Verification items for the finished model (mm, model axes). Face numbers are marked on the shaded views. A direction names the side the tool comes from. Give positions to 0.01 mm unless a question says otherwise; leave off trailing zeros. Write each loop counter-clockwise with the first axis right and the second up, starting at its lowest first coordinate (ties: lowest second). Pieces come first, ordered by that corner, then holes. Notation, with made-up numbers: (40, -20.5) - (57, -20.5) arc R9 cw to (57, -15.5) - close; hole circle Ø6 at (69, 38). An arc over 180 degrees is marked (long way). Answer as a JSON object with one key per item and string values. Group by question number.
Item 1: Sectioned sample at C-C, the plane y = -4.75. Record the boundary of the cut face in (x, z).
Item 2: Draft check along Y on the marked faces 4, 5, 6 and 7. Enter one of: +Y half, -Y half, draft (parallel to the pull), parting line (faces both ways), or undercut.
Item 3: Sectioned sample at A-A, the plane x = -9. Record the boundary of the cut face in (y, z).
Item 4: Sectioned sample at B-B, the plane z = 33. Record the boundary of the cut face in (x, y), and give its area (3 significant figures).
Item 5: Tool access check on the marked faces 1, 2 and 3. Record the directions out of +Z, -Z, +X, -X, +Y, -Y that give a thin tool (end or side, any length) a straight path to the whole face; none if there is none.
Item 6: Scan lines: line 1 along X through (y, z) = (-1.25, 44.5); line 2 along Y through (x, z) = (-0.5, 53.5); line 3 along X through (y, z) = (-7.25, 35). Record each from-to range of solid material in increasing order. Write a range as [from, to].
Item 7: Go/stop test with flat-tipped pins: pin 1 (0.9 mm diameter, centred on y = 8, z = 33.5, fed in from -X); pin 2 (0.9 mm diameter, centred on y = 8.5, z = 37, fed in from +X). Record where each tip stops, or that it passes through.
Item 8: Sectioned sample at D-D, the plane z = 53. Record the boundary of the cut face in (x, y).
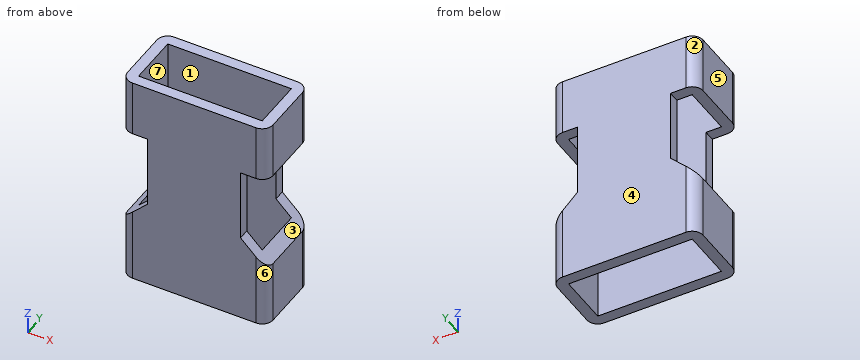
```python
from build123d import *

# Parameters (mm, degrees)
F0_W     = 34
F0_H     = 14
F1_DEPTH = 60
F3_DEPTH = 12.5


with BuildPart() as f1:
    # F0 (on Top) → F1 (new body)
    with BuildSketch(Plane.XY):
        with BuildLine():
            Line((-17, -10), (17, -10))
            ThreePointArc((17, -10), (19.12132, -9.12132), (20, -7))
            Line((20, -7), (20, 7))
            ThreePointArc((20, 7), (19.12132, 9.12132), (17, 10))
            Line((17, 10), (-17, 10))
            ThreePointArc((-17, 10), (-19.12132, 9.12132), (-20, 7))
            Line((-20, 7), (-20, -7))
            ThreePointArc((-20, -7), (-19.12132, -9.12132), (-17, -10))
        make_face()
        Rectangle(F0_W, F0_H, mode=Mode.SUBTRACT)
    extrude(amount=F1_DEPTH)

    # F2 (on Front) → F3 (cut, symmetric)
    with BuildSketch(Plane.XZ):
        Polygon((-25.043013, 44.406913), (-22.849802, 14.579257), (-12.761037, 24.448702), (-12.761037, 44.406913), align=None)
        Polygon((22.849802, 14.579257), (25.043013, 44.406913), (12.761037, 44.406913), (12.761037, 24.448702), align=None)
    extrude(amount=F3_DEPTH, both=True, mode=Mode.SUBTRACT)


solid = f1.part
```
Geometry check:
{
 "1": {"outline": "(-20, 0) - (-17, 0) - (-17, 20.3) - (-20, 17.37) - close; (-20, 44.41) - (-17, 44.41) - (-17, 60) - (-20, 60) - close; (17, 0) - (20, 0) - (20, 17.37) - (17, 20.3) - close; (17, 44.41) - (20, 44.41) - (20, 60) - (17, 60) - close"},
 "2": {"face 4": "+Y half", "face 5": "draft", "face 6": "-Y half", "face 7": "undercut"},
 "3": {"outline": "(-10, 0) - (-7, 0) - (-7, 60) - (-10, 60) - close; (7, 0) - (10, 0) - (10, 60) - (7, 60) - close"},
 "4": {"outline": "(-12.76, -10) - (12.76, -10) - (12.76, -7) - (-12.76, -7) - close; (-12.76, 7) - (12.76, 7) - (12.76, 10) - (-12.76, 10) - close", "area": "153 mm^2"},
 "5": {"face 1": "+Z, -Z", "face 2": "+Z, -Z, -X, +Y", "face 3": "+X, +Y, -Y"},
 "6": {"line 1": "[-20, -17], [17, 20]", "line 2": "[-10, -7], [7, 10]", "line 3": "[-12.76, 12.76]"},
 "7": {"pin 1": "x = -12.76", "pin 2": "x = 12.76"},
 "8": {"outline": "(-20, -7) arc R3 ccw to (-17, -10) - (17, -10) arc R3 ccw to (20, -7) - (20, 7) arc R3 ccw to (17, 10) - (-17, 10) arc R3 ccw to (-20, 7) - close; hole (-17, -7) - (17, -7) - (17, 7) - (-17, 7) - close"}
}
